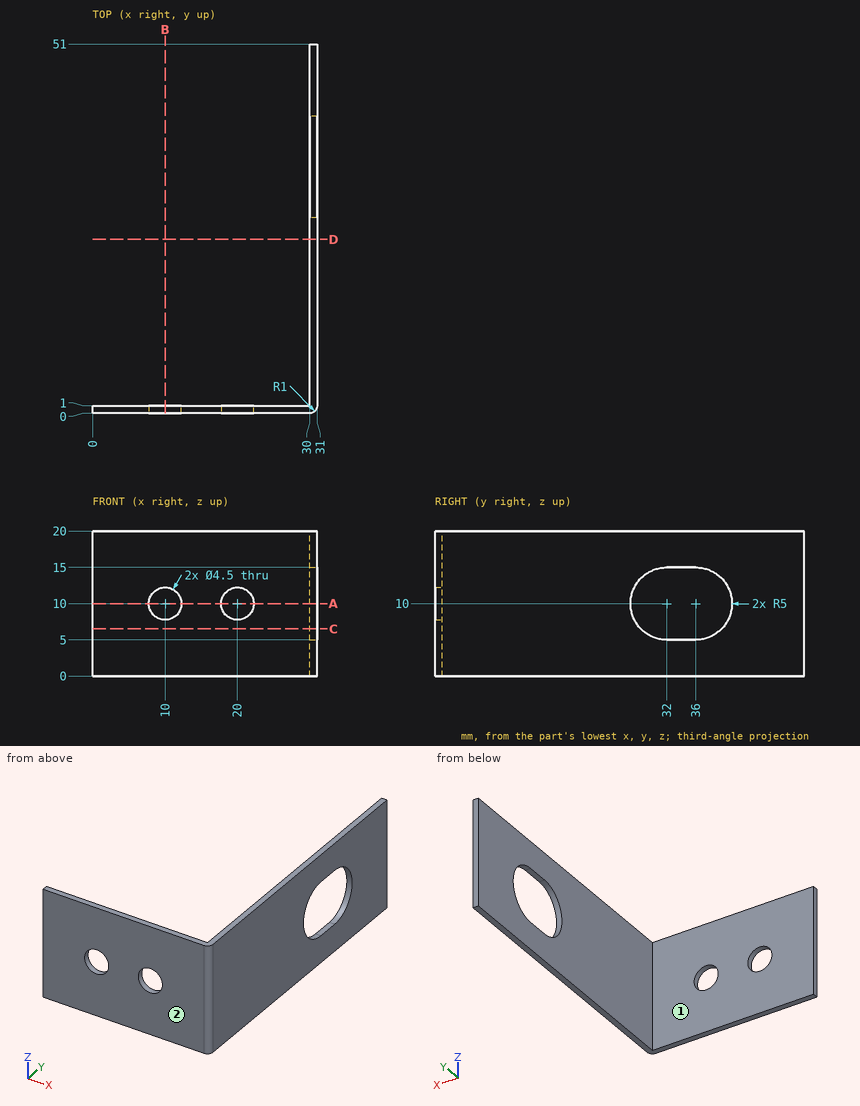
Answer from the drawing. Dimensions are ordinates in mm from the lowest x, y and z of the part. A direction names the side the tool comes from. Give positions to 0.01 mm unless a question says otherwise; leave off trailing zeros. Order: outer loops, then holes, each group sorted by start corner. A loop starts at its lowest first (then second) coordinate and runs counter-clockwise, first axis right, second up.
(1) Given pin 1 (3 mm diameter, centred on y = 20.5, z = 2.5, fed in from -X); pin 2 (5 mm diameter, centred on x = 20, z = 10, fed in from +Y), each flat-ended and moving along its own axis, determine where each tip first touches the part or whether it passes through.
(2) Find section A-A (z = 10). Give the vertices of the cut face in (x, y).
(3) Straight lines are drawn through the part: L1, parallel to Z at x = 10, y = 0.35; L2, parallel to X at y = 15, z = 7.75; L3, parallel to Y at x = 23.5, z = 7. For each, find the intervals that lie inside material, in ascending order.
(4) Find section D-D (y = 24). Give the vertices of the cut face in (x, z), plus the area to 3 significant figures.
(5) Find section B-B (x = 10). Give the vertices of the cut face in (y, z), plus the area to 3 significant figures.
(6) For the marked faces 1 and 2, determine the directions among +Z, -Z, +X, -X, +Y, -Y from which every point of the face is accessible in a straight line to the end or side of a thin tool.
(7) Find section C-C (z = 6.5). Give the vertices of the cut face in (x, y), plus the area to 3 significant figures.
Result sheet:
1. pin 1: stops at x = 30
1. pin 2: stops at y = 1
2. outline: (0, 0) - (7.75, 0) - (7.75, 1) - (0, 1) - close; (12.25, 0) - (17.75, 0) - (17.75, 1) - (12.25, 1) - close; (22.25, 0) - (30, 0) arc R1 ccw to (31, 1) - (31, 27) - (30, 27) - (30, 1) - (22.25, 1) - close; (30, 41) - (31, 41) - (31, 51) - (30, 51) - close
3. L1: z = 0 to 7.75, 12.25 to 20
3. L2: x = 30 to 31
3. L3: y = 0 to 1
4. outline: (30, 0) - (31, 0) - (31, 20) - (30, 20) - close
4. area: 20.0 mm2
5. outline: (0, 0) - (1, 0) - (1, 7.75) - (0, 7.75) - close; (0, 12.25) - (1, 12.25) - (1, 20) - (0, 20) - close
5. area: 15.5 mm2
6. face 1: +Z, -Z, -X, +Y
6. face 2: +Z, -Z, +X, -X, -Y
7. outline: (0, 0) - (30, 0) arc R1 ccw to (31, 1) - (31, 28.43) - (30, 28.43) - (30, 1) - (0, 1) - close; (30, 39.57) - (31, 39.57) - (31, 51) - (30, 51) - close
7. area: 69.6 mm2
